Read the model definition and answer for the solid it produces. Units are mm, in the model's axes. A direction names the side the tool comes from. Coordinates: 2 decimals unless noted, no trailing zeros. Loops run counter-clockwise (first coordinate to the right, second up) from the corner with the lowest first, then second, coordinate; pieces in that order, holes last. Notation, with made-up numbers: (35.25, 59.25) - (82.25, 59.25) arc R19 cw to (82.25, 68.25) - close; hole circle Ø3 at (-26, -40). An arc over 180 degrees is marked (long way). Use one line per item in the form item = value.
from build123d import *

# Parameters (mm, degrees)
CYLINDER004_R             = 1.9
CYLINDER004_DEPTH         = 15
BOX005_W                  = 15
BOX005_H                  = 3.4
BOX005_DEPTH              = 17
ARRAY001_Y_COUNT          = 3
ARRAY001_Y_PITCH          = 6
CYLINDER003_R             = 7.5
CYLINDER003_DEPTH         = 15
BOX004_W                  = 15
BOX004_H                  = 15
BOX004_DEPTH              = 12.5
BOX003_W                  = 15
BOX003_H                  = 3.4
BOX003_DEPTH              = 17
ARRAY_Y_COUNT             = 2
ARRAY_Y_PITCH             = 6
CYLINDER002_R             = 2.2
CYLINDER002_DEPTH         = 6
CYLINDER001_R             = 1.9
CYLINDER001_DEPTH         = 15
FUSION001_PLACEMENT_ANGLE = 90
CYLINDER_R                = 7.5
CYLINDER_DEPTH            = 19.6
BOX002_W                  = 15
BOX002_H                  = 19.6
BOX002_DEPTH              = 12.5
BODY009_PLACEMENT_ANGLE   = 180
BOX012_W                  = 15
BOX012_H                  = 15
BOX012_DEPTH              = 30
FILLET003_1_R             = 3
FILLET003_2_R             = 2
FILLET003_3_R             = 0.5


with BuildPart() as side_2_bolt_hole:
    # Cylinder004 → Cylinder004 (new body)
    with BuildSketch(Plane(origin=(0, 7.5, 12.5), x_dir=(1, 0, 0), z_dir=(0, -1, 0))):
        Circle(CYLINDER004_R)
    extrude(amount=CYLINDER004_DEPTH)


with BuildPart() as side_2_extract_fusion:
    # Box005 → Box005 (new body)
    with BuildSketch(Plane(origin=(-7.5, -7.7, 3), x_dir=(1, 0, 0), z_dir=(0, 0, 1))):
        with Locations((7.5, 1.7)):
            Rectangle(BOX005_W, BOX005_H)
    extrude(amount=BOX005_DEPTH)

    # Array001 Y: side 2 extract fusion ×3


with BuildPart() as side_2_extract_fusion_1:
    add(side_2_extract_fusion.part)
    with Locations(*[(0, i * ARRAY001_Y_PITCH, 0) for i in range(1, ARRAY001_Y_COUNT)]):
        add(side_2_extract_fusion.part)

    # Fusion004: union side 2 bolt hole
    add(side_2_bolt_hole.part)


with BuildPart() as outer_cylinder001:
    # Cylinder003 → Cylinder003 (new body)
    with BuildSketch(Plane(origin=(0, 7.5, 12.5), x_dir=(1, 0, 0), z_dir=(0, -1, 0))):
        Circle(CYLINDER003_R)
    extrude(amount=CYLINDER003_DEPTH)


with BuildPart() as side_2_cut_clone003:
    # Box004 → Box004 (new body)
    with BuildSketch(Plane(origin=(-7.5, -7.5, 0), x_dir=(1, 0, 0), z_dir=(0, 0, 1))):
        with Locations((7.5, 7.5)):
            Rectangle(BOX004_W, BOX004_H)
    extrude(amount=BOX004_DEPTH)

    # Fusion003: union outer cylinder001
    add(outer_cylinder001.part)

    # Cut001: cut side 2 extract fusion
    add(side_2_extract_fusion_1.part, mode=Mode.SUBTRACT)


with BuildPart() as side_2_cut_clone003_1:
    # Body008 placement: moved
    add(side_2_cut_clone003.part.moved(Location((0, 0, 30))))


with BuildPart() as side_3_extract_cube_array:
    # Box003 → Box003 (new body)
    with BuildSketch(Plane(origin=(-7.5, -7.7, 3), x_dir=(1, 0, 0), z_dir=(0, 0, 1))):
        with Locations((7.5, 1.7)):
            Rectangle(BOX003_W, BOX003_H)
    extrude(amount=BOX003_DEPTH)

    # Array Y: side 3 extract cube array ×2


with BuildPart() as side_3_extract_cube_array_1:
    add(side_3_extract_cube_array.part)
    with Locations(*[(0, i * ARRAY_Y_PITCH, 0) for i in range(1, ARRAY_Y_COUNT)]):
        add(side_3_extract_cube_array.part)


with BuildPart() as side_3_extract_cube_array_2:
    # Array placement: moved
    add(side_3_extract_cube_array_1.part.moved(Location((0, 3, 0))))


with BuildPart() as insert_hole:
    # Cylinder002 → Cylinder002 (new body)
    with BuildSketch(Plane.XY):
        Circle(CYLINDER002_R)
    extrude(amount=CYLINDER002_DEPTH)


with BuildPart() as side_3_extract_fusion:
    # Cylinder001 → Cylinder001 (new body)
    with BuildSketch(Plane.XY.offset(6)):
        Circle(CYLINDER001_R)
    extrude(amount=CYLINDER001_DEPTH)

    # Fusion001: union insert hole
    add(insert_hole.part)


with BuildPart() as side_3_extract_fusion_1:
    # Fusion001 placement: moved
    add(side_3_extract_fusion.part.moved(Location((0, 11.1, 12.5))).rotate(Axis((0, 11.1, 12.5), (1, 0, 0)), FUSION001_PLACEMENT_ANGLE))

    # Fusion002: union side 3 extract cube array
    add(side_3_extract_cube_array_2.part)


with BuildPart() as outer_cylinder:
    # Cylinder → Cylinder (new body)
    with BuildSketch(Plane(origin=(0, 11.1, 12.5), x_dir=(1, 0, 0), z_dir=(0, -1, 0))):
        Circle(CYLINDER_R)
    extrude(amount=CYLINDER_DEPTH)


with BuildPart() as side_3_cut_clone003:
    # Box002 → Box002 (new body)
    with BuildSketch(Plane(origin=(-7.5, -8.5, 0), x_dir=(1, 0, 0), z_dir=(0, 0, 1))):
        with Locations((7.5, 9.8)):
            Rectangle(BOX002_W, BOX002_H)
    extrude(amount=BOX002_DEPTH)

    # Fusion: union outer cylinder
    add(outer_cylinder.part)

    # Cut: cut side 3 extract fusion
    add(side_3_extract_fusion_1.part, mode=Mode.SUBTRACT)


with BuildPart() as side_3_cut_clone003_1:
    # Body009 placement: moved
    add(side_3_cut_clone003.part.rotate(Axis((0, 0, 0), (0, 1, 0)), BODY009_PLACEMENT_ANGLE))


with BuildPart() as obj1:
    # Box012 → Box012 (new body)
    with BuildSketch(Plane(origin=(-7.5, -7.5, 0), x_dir=(1, 0, 0), z_dir=(0, 0, 1))):
        with Locations((7.5, 7.5)):
            Rectangle(BOX012_W, BOX012_H)
    extrude(amount=BOX012_DEPTH)

    # Fusion010: union side 2 cut clone003, side 3 cut clone003
    add(side_2_cut_clone003_1.part)
    add(side_3_cut_clone003_1.part)

    # Fillet003 1
    fillet003_1_edges = [obj1.edges().sort_by_distance(p)[0] for p in [
        (0, 11.1, 0),
    ]]
    fillet(fillet003_1_edges, radius=FILLET003_1_R)

    # Fillet003 2
    fillet003_2_edges = [obj1.edges().sort_by_distance(p)[0] for p in [
        (0, -7.5, 33),
        (0, 7.5, 33),
    ]]
    fillet(fillet003_2_edges, radius=FILLET003_2_R)

    # Fillet003 3
    fillet003_3_edges = [obj1.edges().sort_by_distance(p)[0] for p in [
        (0, -8.5, 0),
    ]]
    fillet(fillet003_3_edges, radius=FILLET003_3_R)


solid = obj1.part
Item 1: The part is cut by section B-B on z = -7. Give the vertices of the cut face in (x, y).
Results below:
outline = (-7.5, -8.5) - (7.5, -8.5) - (7.5, -4.7) - (-7.5, -4.7) - close; (-7.5, -1.3) - (7.5, -1.3) - (7.5, 1.3) - (-7.5, 1.3) - close; (-7.5, 4.7) - (7.5, 4.7) - (7.5, 11.1) - (-7.5, 11.1) - close
Item 2: Which of the six approach directions +Z, -Z, +X, -X, +Y, -Y give full straight-line access (tool end or side, diameter ignored) to faces 1 (the flat face through (0, 4.7, -9)), 2 (the flat face through (0, 7.5, 15)), 3 (the flat face through (0, -5, 33))?
Results below:
face_1 = -Z, +X, -X
face_2 = +Z, +X, -X, +Y
face_3 = +Z, +X, -X, -Y
Item 3: For a pull along X with two mould halves and no side action, classify faces 4 (the cylindrical face through (0.412, 0.018, -10.645)), 5 (the flat face through (0, -3, -3)), 6 (the flat face through (-7.5, 1, 9)) as +X half, -X half, draft (parallel to the pull), parting line (faces both ways), or undercut.
Results below:
face_4 = undercut
face_5 = draft
face_6 = -X half
Item 4: Each of these flat-tipped pins is pushed along its axis until it touches: P1, Ø4.5, axis at x = 1.5, z = 39, coming from the -Y side; P2, Ø3, axis at x = 0, z = -12.5, coming from the +Y side; P3, Ø7.5, axis at x = 3.5, z = 15, coming from the +Y side; P4, Ø2, axis at x = -5, z = 19, coming from the -Y side. Where does it stop, or does it pass through?
Results below:
P1 = -4.3
P2 = through
P3 = 7.5
P4 = -7.5
Item 5: Find the intervals of material crossed by L1, parallel to Y at x = -1.25, z = -4; L2, parallel to Y at x = 6.5, z = 34; L3, parallel to Z at x = 0, y = 0.5, in increasing order.
Results below:
L1 = -8.5 to -4.7, -1.3 to 1.3, 4.7 to 11.1
L2 = -4.3 to -1.7, 1.7 to 4.3
L3 = -20 to -14.4, -10.6 to 33
Item 6: The part is cut by section A-A on z = 36. Give the vertices of the cut face in (x, y), plus the area to 3 significant figures.
Results below:
outline = (-7.5, -4.3) - (7.5, -4.3) - (7.5, -1.7) - (-7.5, -1.7) - close; (-7.5, 1.7) - (7.5, 1.7) - (7.5, 4.3) - (-7.5, 4.3) - close
area = 78.0 mm²
Item 7: The part is cut by section D-D on y = -6.75. Give the vertices of the cut face in (x, z).
Results below:
outline = (-7.5, -12.5) arc R7.5 ccw to (7.5, -12.5) - (7.5, 32.56) - (-7.5, 32.56) - close; hole circle Ø3.8 at (0, -12.5)
Item 8: The part is cut by section C-C on x = 0. Count the separate pieces of the cut face and the enclosed holes in it, plus the area to 3 significant figures.
Results below:
separate_pieces = 6
enclosed_holes = 0
area = 784 mm²
